from build123d import *

# Parameters (mm, degrees)
F0_R     = 11.708772
F0_R_2   = 12.511631
F1_DEPTH = 87.884


with BuildPart() as f1:
    # F0 (on Top) → F1 (new body)
    with BuildSketch(Plane.XY):
        with BuildLine():
            ThreePointArc((-60.466758, 32.941471), (-36.576779, 29.201541), (-23.419007, 49.489252))
            ThreePointArc((-23.419007, 49.489252), (-24.717173, 56.972833), (-28.459983, 63.581963))
            ThreePointArc((-28.459983, 63.581963), (-59.487612, 66.864763), (-63.20755, 35.886503))
            Line((-63.20755, 35.886503), (-60.466758, 32.941471))
        make_face()
        with Locations((-45.638505, 49.489252)):
            Circle(F0_R, mode=Mode.SUBTRACT)
        with BuildLine():
            ThreePointArc((-28.459983, 63.581963), (-24.717173, 56.972833), (-23.419007, 49.489252))
            ThreePointArc((-23.419007, 49.489252), (-36.576779, 29.201541), (-60.466758, 32.941471))
            Line((-60.466758, 32.941471), (-28.93399, -0.941065))
            ThreePointArc((-28.93399, -0.941065), (-25.211548, 31.012543), (6.954043, 30.498322))
            Line((6.954043, 30.498322), (-28.459983, 63.581963))
        make_face()
        with BuildLine():
            ThreePointArc((-63.20755, 35.886503), (-61.903945, 34.351828), (-60.466758, 32.941471))
            Line((-60.466758, 32.941471), (-63.20755, 35.886503))
        make_face()
        with BuildLine():
            ThreePointArc((14.562543, 12.978454), (12.578309, 22.528782), (6.954043, 30.498322))
            ThreePointArc((6.954043, 30.498322), (-25.211548, 31.012543), (-28.93399, -0.941065))
            Line((-28.93399, -0.941065), (-24.697207, -5.493566))
            ThreePointArc((-24.697207, -5.493566), (0.794317, -8.71569), (14.562543, 12.978454))
        make_face()
        with Locations((-9.412947, 12.978454)):
            Circle(F0_R_2, mode=Mode.SUBTRACT)
        with BuildLine():
            Line((-24.697207, -5.493566), (-28.93399, -0.941065))
            ThreePointArc((-28.93399, -0.941065), (-26.963833, -3.35527), (-24.697207, -5.493566))
        make_face()
    extrude(amount=-F1_DEPTH)


solid = f1.part
The listing builds one solid part. Answer for the finished solid, in the listing's coordinates (mm). Coordinates: 2 decimals unless noted, no trailing zeros. Write each loop counter-clockwise with the first axis right and the second up, starting at its lowest first coordinate (ties: lowest second). Pieces come first, ordered by that corner, then holes. Notation, with made-up numbers: M -34,76.5 L -22,76.5 A25 cw -22,98.5 Z; hole C 4.25,59.25 d4. An arc over 180 degrees is marked long. Put each result on its own line as item: value. Start each with the question number.
1. A cutting plane is placed at D-D on y = -3. Write down the section's boundary in (x, z).
2. Consider line 1 (X direction, y = 42, z = -41); line 2 (Y direction, x = -17.5, z = -56); line 3 (X direction, y = 11, z = -4). Determine where each line is inside the solid, lowest interval first. Write a range as from..to.
3. Flat-ended cylindrical pins translate along their axes: P1, Ø10, axis at y = 48.5, z = -14.5, coming from the +X side; P2, Ø5, axis at x = -16, z = -51.5, coming from the +Y side; P3, Ø1, axis at y = 30.5, z = -17, coming from the -X side. Find the tip coordinate at first contact, or state that the pin passes through.
4. A cutting plane is placed at A-A on y = 45. Write down the section's boundary in (x, z), then the cut area to 3 significant figures.
5. A cutting plane is placed at B-B on x = -55.5. Write down the section's boundary in (y, z), then the cut area to 3 significant figures.
6. A cutting plane is placed at C-C on z = -60. Write down the section's boundary in (x, y), then the cut area to 3 significant figures.
7. For a pull along X with two mould halves and no side action, classify faces 1 (the cylindrical face through (-54.93, 42.365, -43.327)), 2 (the flat face through (-27, 31, 0)), 3 (the flat face through (-10.505, 46.809, -43.327)), 4 (the cylindrical face through (-19.342, 5.365, -43.327)) as pulls with the +X half, pulls with the -X half, needs draft (parallel to the pull), parting line crosses it, or undercut.
Resolved:
1. outline: M -27.29,-87.88 L 8.46,-87.88 L 8.46,0 L -27.29,0 Z
2. line 1: x = -66.56..-54.64, -36.64..-5.36
2. line 2: y = -9.59..3.43, 22.53..53.34
2. line 3: x = -40.05..-21.77, 2.94..14.48
3. P1: stops at x = -6.96
3. P2: stops at y = 54.28
3. P3: stops at x = -58.66
4. outline: M -67.4,-87.88 L -56.45,-87.88 L -56.45,0 L -67.4,0 Z; M -34.82,-87.88 L -8.57,-87.88 L -8.57,0 L -34.82,0 Z
4. area: 3,270 mm2
5. outline: M 27.6,-87.88 L 43.18,-87.88 L 43.18,0 L 27.6,0 Z; M 55.8,-87.88 L 69.4,-87.88 L 69.4,0 L 55.8,0 Z
5. area: 2,560 mm2
6. outline: M -63.21,35.89 A22.22 ccw -60.47,32.94 L -28.93,-0.94 A23.98 ccw -24.7,-5.49 A23.98 ccw 14.56,12.98 A23.98 ccw 6.95,30.5 L -28.46,63.58 A22.22 ccw Z; hole C -45.64,49.49 d23.42; hole C -9.41,12.98 d25.02
6. area: 3,120 mm2
7. face 1: undercut
7. face 2: needs draft
7. face 3: pulls with the +X half
7. face 4: undercut
